```python
from build123d import *

# Parameters (mm, degrees)
F0_W     = 25.4
F0_H     = 100
F0_R     = 2.6
F1_DEPTH = 6.35


with BuildPart() as f1:
    # F0 (on Front) → F1 (new body)
    with BuildSketch(Plane.XZ):
        Rectangle(F0_W, F0_H)
        with Locations((-6.35, -40)):
            Circle(F0_R, mode=Mode.SUBTRACT)
        with Locations((6.35, -40)):
            Circle(F0_R, mode=Mode.SUBTRACT)
        with Locations((-6.35, 20)):
            Circle(F0_R, mode=Mode.SUBTRACT)
        with Locations((-6.35, 40)):
            Circle(F0_R, mode=Mode.SUBTRACT)
        with Locations((6.35, 20)):
            Circle(F0_R, mode=Mode.SUBTRACT)
        with Locations((6.35, 40)):
            Circle(F0_R, mode=Mode.SUBTRACT)
    extrude(amount=F1_DEPTH)


solid = f1.part
```
Verification items for the finished model (mm, model axes). Coordinates: 2 decimals unless noted, no trailing zeros. Loops run counter-clockwise (first coordinate to the right, second up) from the corner with the lowest first, then second, coordinate; pieces in that order, holes last. Notation, with made-up numbers: (-25, -20.5) -> (0, -20.5) arc R22 cw to (0, 18.5) -> close; hole circle Ø3 at (9, 61). An arc over 180 degrees is marked (long way). Answer in a Markdown table with one row per item. Add a question column.
1. Material ranges on probe 1 along Z at (x, y) = (6.35, -3); probe 2 along Z at (x, y) = (-5, -5.5); probe 3 along X at (y, z) = (-0.75, -38), recorded low to high. Write a range as [from, to].
2. Section check A-A, the plane y = -3.5. Enter the section's corners in (x, z).
3. Section check C-C, the plane x = 6.35. Enter the section's corners in (y, z).
4. Section check B-B, the plane z = -40. Enter the section's corners in (x, y), then the cut area to 4 significant figures.
5. Draft check along Z on faces 1 (the face through (0, -3, 50)), 2 (the face through (5.79, -3.13, -42.54)), 3 (the face through (12.7, -3, -1)). Enter one of: +Z half, -Z half, draft (parallel to the pull), parting line (faces both ways), or undercut.
6. Section check D-D, the plane x = -8. Enter the section's corners in (y, z).
Derived:
| question | item | result |
|---|---|---|
| 1 | probe 1 | z = [-50, -42.6], [-37.4, 17.4], [22.6, 37.4], [42.6, 50] |
| 1 | probe 2 | z = [-50, -42.22], [-37.78, 17.78], [22.22, 37.78], [42.22, 50] |
| 1 | probe 3 | x = [-12.7, -8.01], [-4.69, 4.69], [8.01, 12.7] |
| 2 | outline | (-12.7, -50) -> (12.7, -50) -> (12.7, 50) -> (-12.7, 50) -> close; hole circle Ø5.2 at (-6.35, -40); hole circle Ø5.2 at (-6.35, 20); hole circle Ø5.2 at (-6.35, 40); hole circle Ø5.2 at (6.35, -40); hole circle Ø5.2 at (6.35, 20); hole circle Ø5.2 at (6.35, 40) |
| 3 | outline | (-6.35, -50) -> (0, -50) -> (0, -42.6) -> (-6.35, -42.6) -> close; (-6.35, -37.4) -> (0, -37.4) -> (0, 17.4) -> (-6.35, 17.4) -> close; (-6.35, 22.6) -> (0, 22.6) -> (0, 37.4) -> (-6.35, 37.4) -> close; (-6.35, 42.6) -> (0, 42.6) -> (0, 50) -> (-6.35, 50) -> close |
| 4 | outline | (-12.7, -6.35) -> (-8.95, -6.35) -> (-8.95, 0) -> (-12.7, 0) -> close; (-3.75, -6.35) -> (3.75, -6.35) -> (3.75, 0) -> (-3.75, 0) -> close; (8.95, -6.35) -> (12.7, -6.35) -> (12.7, 0) -> (8.95, 0) -> close |
| 4 | area | 95.25 mm² |
| 5 | face 1 | +Z half |
| 5 | face 2 | undercut |
| 5 | face 3 | draft |
| 6 | outline | (-6.35, -50) -> (0, -50) -> (0, -42.01) -> (-6.35, -42.01) -> close; (-6.35, -37.99) -> (0, -37.99) -> (0, 17.99) -> (-6.35, 17.99) -> close; (-6.35, 22.01) -> (0, 22.01) -> (0, 37.99) -> (-6.35, 37.99) -> close; (-6.35, 42.01) -> (0, 42.01) -> (0, 50) -> (-6.35, 50) -> close |
